Verification items for the finished model (mm, model axes). Face numbers are marked on the shaded views. A direction names the side the tool comes from. Coordinates: 2 decimals unless noted, no trailing zeros. Write each loop counter-clockwise with the first axis right and the second up, starting at its lowest first coordinate (ties: lowest second). Pieces come first, ordered by that corner, then holes. Notation, with made-up numbers: (-20, 29) -> (-5, 29) arc R24 ccw to (-5, 49) -> close; hole circle Ø8 at (-21.5, 19.5). An arc over 180 degrees is marked (long way). Use CSV: the item, a comma, the result in double quotes.
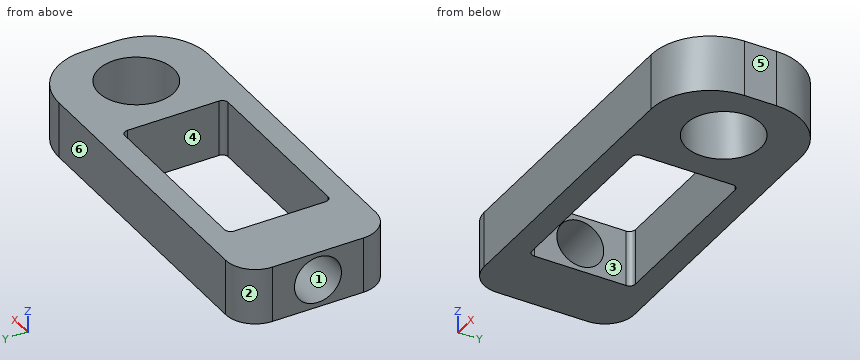
```python
from build123d import *

# Parameters (mm, degrees)
SKETCH1_W           = 63.5
SKETCH1_H           = 25.4
BOSS_EXTRUDE1_DEPTH = 9.525
SKETCH5_R           = 6.35
SKETCH5_W           = 31
SKETCH5_H           = 17.5
CUT_EXTRUDE3_DEPTH  = 10.525
CUT_EXTRUDE2_REACH  = 65.5
SKETCH4_R           = 3.9751
FILLET4_R           = 10
FILLET5_R           = 5
FILLET6_R           = 1


with BuildPart() as part:
    # Sketch1 → Boss-Extrude1 (new body)
    with BuildSketch(Plane.XY):
        with Locations((31.75, 12.7)):
            Rectangle(SKETCH1_W, SKETCH1_H)
    extrude(amount=BOSS_EXTRUDE1_DEPTH)

    # Sketch5 → Cut-Extrude3 (cut, through all)
    with BuildSketch(Plane.XY.offset(9.525)):
        with Locations((52.803125, 12.7)):
            Circle(SKETCH5_R)
        with Locations((26.60625, 12.7)):
            Rectangle(SKETCH5_W, SKETCH5_H)
    extrude(amount=-CUT_EXTRUDE3_DEPTH, mode=Mode.SUBTRACT)

    # Sketch4 → Cut-Extrude2 (cut, up to next)
    with BuildSketch(Plane.ZY, mode=Mode.PRIVATE) as cut_extrude2_sk1:
        with Locations((4.7625, 12.7)):
            Circle(SKETCH4_R)
    cut_extrude2_tool1 = extrude(cut_extrude2_sk1.sketch, amount=-CUT_EXTRUDE2_REACH, mode=Mode.PRIVATE) & part.part
    add(cut_extrude2_tool1.solids().sort_by_distance((0, 12.7, 4.7625))[0], mode=Mode.SUBTRACT)

    # Fillet4
    fillet4_edges = [part.edges().sort_by_distance(p)[0] for p in [
        (63.5, 25.4, 4.7625),
        (63.5, 0, 4.7625),
    ]]
    fillet(fillet4_edges, radius=FILLET4_R)

    # Fillet5
    fillet5_edges = [part.edges().sort_by_distance(p)[0] for p in [
        (0, 25.4, 4.7625),
        (0, 0, 4.7625),
    ]]
    fillet(fillet5_edges, radius=FILLET5_R)

    # Fillet6
    fillet6_edges = [part.edges().sort_by_distance(p)[0] for p in [
        (42.10625, 21.45, 4.7625),
        (42.10625, 3.95, 4.7625),
        (11.10625, 3.95, 4.7625),
        (11.10625, 21.45, 4.7625),
    ]]
    fillet(fillet6_edges, radius=FILLET6_R)


solid = part.part
```
1) Cross-section at C-C (z = 3.25). Record the boundary of the cut face in (x, y), plus the area to 3 significant figures.
Return value:
outline,"(0, 5) arc R5 ccw to (5, 0) -> (53.5, 0) arc R10 ccw to (63.5, 10) -> (63.5, 15.4) arc R10 ccw to (53.5, 25.4) -> (5, 25.4) arc R5 ccw to (0, 20.4) -> (0, 16.38) -> (11.11, 16.38) -> (11.11, 20.45) arc R1 cw to (12.11, 21.45) -> (41.11, 21.45) arc R1 cw to (42.11, 20.45) -> (42.11, 4.95) arc R1 cw to (41.11, 3.95) -> (12.11, 3.95) arc R1 cw to (11.11, 4.95) -> (11.11, 9.02) -> (0, 9.02) -> close; hole circle Ø12.7 at (52.8, 12.7)"
area,"809 mm2"
2) Cross-section at D-D (x = 57). Record the boundary of the cut face in (y, z) (1 decimal).
Return value:
outline,"(0.6, 0) -> (7.9, 0) -> (7.9, 9.5) -> (0.6, 9.5) -> close; (17.5, 0) -> (24.8, 0) -> (24.8, 9.5) -> (17.5, 9.5) -> close"
3) Set-up check for the marked faces 1, 2 and 3: record each of +Z, -Z, +X, -X, +Y, -Y from which the full face is reachable in a straight line by a thin tool's end or side.
Return value:
face 1,"-X"
face 2,"+Z, -Z, -X, +Y"
face 3,"+Z, -Z"
4) Mould release check, pull along Y, two halves, no side actions. Record for the marked faces 4, 5 and 6: released by +Y, released by -Y, zero draft, split by the parting line, or undercut.
Return value:
face 4,"undercut"
face 5,"zero draft"
face 6,"released by +Y"
5) Scan lines: L1, parallel to Y at x = 36.5, z = 5; L2, parallel to X at y = 8, z = 4; L3, parallel to X at y = 12.75, z = 1. Record each from-to range of solid material in increasing order.
Return value:
L1,"0 to 3.95, 21.45 to 25.4"
L2,"0 to 11.11, 42.11 to 48.53, 57.07 to 63.3"
L3,"42.11 to 46.45, 59.15 to 63.5"
6) Cross-section at A-A (y = 12.7). Record the boundary of the cut face in (x, z) (3 decimals), plus the area to 3 significant figures.
Return value:
outline,"(0, 0) -> (11.106, 0) -> (11.106, 0.787) -> (0, 0.787) -> close; (0, 8.738) -> (11.106, 8.738) -> (11.106, 9.525) -> (0, 9.525) -> close; (42.106, 0) -> (46.453, 0) -> (46.453, 9.525) -> (42.106, 9.525) -> close; (59.153, 0) -> (63.5, 0) -> (63.5, 9.525) -> (59.153, 9.525) -> close"
area,"100 mm2"
7) Gauge pin test, flat end, axial feed: pin 1 (1 mm diameter, centred on y = 6.5, z = 1.5, fed in from +X). Record the tip position at first contact, or that the pin passes through.
Return value:
pin 1,"x = 63.04"
8) Cross-section at B-B (x = 34). Record the boundary of the cut face in (y, z) (3 decimals), plus the area to 3 significant figures.
Return value:
outline,"(0, 0) -> (3.95, 0) -> (3.95, 9.525) -> (0, 9.525) -> close; (21.45, 0) -> (25.4, 0) -> (25.4, 9.525) -> (21.45, 9.525) -> close"
area,"75.2 mm2"
